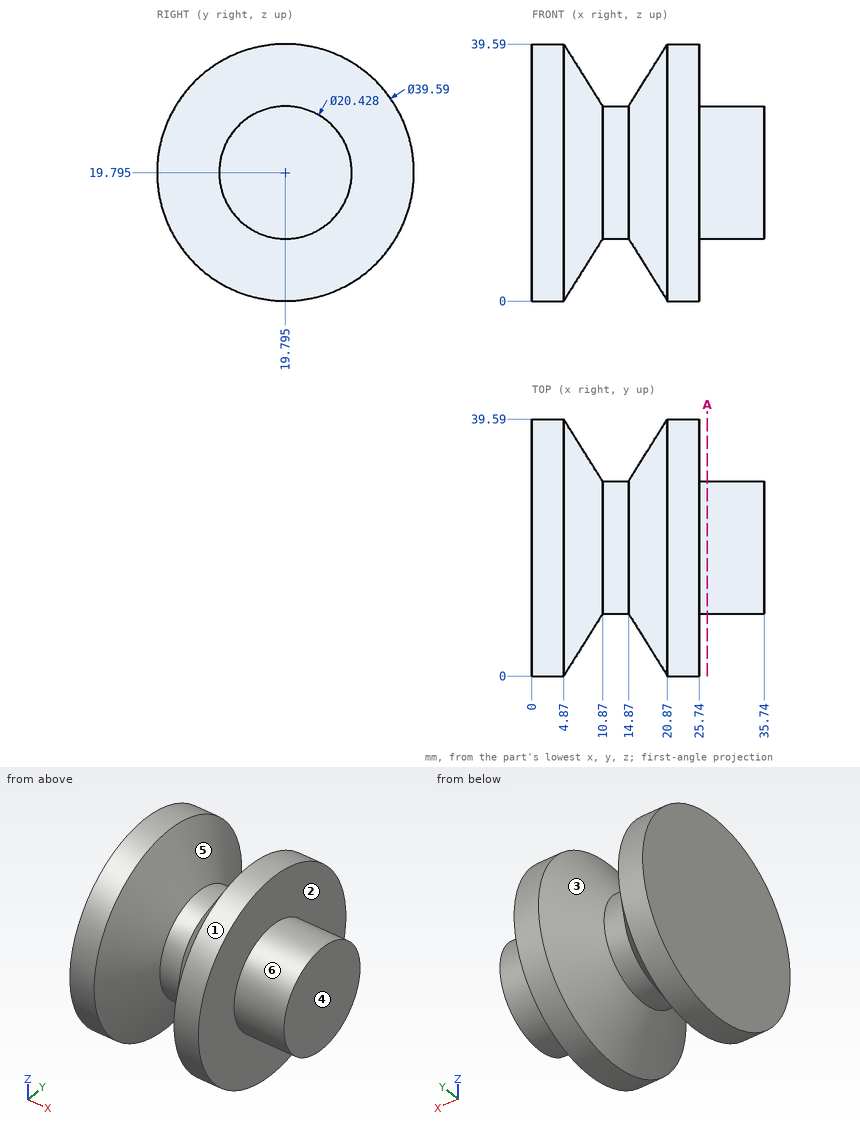
Can you work these out from the drawing? Everything is in mm from the part's minimum corner. A direction names the side the tool comes from. Coordinates: 2 decimals unless noted, no trailing zeros. Loops run counter-clockwise (first coordinate to the right, second up) from the corner with the lowest first, then second, coordinate; pieces in that order, holes last. Notation, with made-up numbers: M 61.5,21 L 73.5,21 A21 ccw 73.5,46 Z; hole C 12,73.5 d10. An arc over 180 degrees is marked long. Put each result on its own line as item: value. Start each with the question number.
(1) I need wall thicknesses on line 1 (X direction, y = 7, z = 26.5); line 2 (X direction, y = 13, z = 11.5); line 3 (Z direction, x = 12, y = 12.5) (1 decimal). Which ranges of each line are inside material? Lowest first, please. Write a range as from..to.
(2) Suppose I cut it at A-A on x = 27. Please give me the cut outline in (y, z) (1 decimal).
(3) Thinking about a two-plate mould opening in X: for the marked faces 4, 5 and 6, which applies, pulls with the +X half, pulls with the -X half, needs draft (parallel to the pull), parting line crosses it, or undercut?
(4) Will these pins go through, and if not, where does the flat tip stop? P1, Ø1.5, axis at x = 27.5, y = 10, coming from the -Z side; P2, Ø6, axis at y = 35, z = 8, coming from the +X side; P3, Ø8, axis at x = 16, z = 8, coming from the +Y side.
(5) For the marked faces 1, 2 and 3, which set-ups out of +Z, -Z, +X, -X, +Y, -Y let a thin tool reach every point of the face, with its end or its side?
Solutions:
1. line 1: x = 0..8.22, 17.52..25.74
1. line 2: x = 0..10.55, 15.19..25.74
1. line 3: z = 12.6..26.9
2. outline: C 19.8,19.8 d20.4
3. face 4: pulls with the +X half
3. face 5: undercut
3. face 6: needs draft
4. P1: stops at z = 15.05
4. P2: stops at x = 25.74
4. P3: stops at y = 34.49
5. face 1: +X, -X
5. face 2: +X
5. face 3: none
